```python
from build123d import *

# Parameters (mm, degrees)
STOCK_SHORT_HANDLE_L_1_START = -1
STOCK_SHORT_HANDLE_L_1_DEPTH = 2
FILLET1_R                    = 0.5


# Read off the part's stored shape, not the designer's step: Stock-short-handle_L-1
with BuildPart() as part:
    # Stock-short-handle_L-1 outline → Stock-short-handle_L-1 (new body)
    with BuildSketch(Plane(origin=(0, 0, 0), x_dir=(1, 0, 0), z_dir=(0, 1, 0)).offset(STOCK_SHORT_HANDLE_L_1_START)):
        with BuildLine():
            Line((5, -39.585762407), (-5, -39.585762407))
            Line((-5, -39.585762407), (-5, -43.585762407))
            ThreePointArc((-5, -43.585762407), (-4.810860404, -44.434752748), (-4.279215401, -45.123165398))
            ThreePointArc((-4.279215401, -45.123165398), (-1.203063357, -47.386267754), (2.120784599, -49.266793861))
            ThreePointArc((2.120784599, -49.266793861), (4.058671148, -49.167239185), (5, -47.470414091))
            Line((5, -47.470414091), (5, -39.585762407))
        make_face()
    extrude(amount=STOCK_SHORT_HANDLE_L_1_DEPTH)

    # Fillet1
    fillet1_edges = [part.edges().sort_by_distance(p)[0] for p in [
        (5, 0, 39.585762407),
        (-5, 0, 39.585762407),
    ]]
    fillet(fillet1_edges, radius=FILLET1_R)


solid = part.part
```
Could you check a few things on this model? Use its own coordinates, in mm. Round coordinates to 2 decimals unless told otherwise and drop trailing zeros. Loops run counter-clockwise (first coordinate to the right, second up) from the corner with the lowest first, then second, coordinate; pieces in that order, holes last. Notation, with made-up numbers: (32, 23.5) -> (80, 23.5) arc R5 ccw to (80, 30.5) -> close; hole circle Ø5 at (83, 12.5). An arc over 180 degrees is marked (long way). Put each result on its own line as item: value.
Q1. I want a section at A-A on y = -0.7. Write out the boundary of the cut face in (x, z), and give its area (3 significant figures).
Checks:
outline: (-5, 40.09) arc R0.5 ccw to (-4.5, 39.59) -> (4.5, 39.59) arc R0.5 ccw to (5, 40.09) -> (5, 47.47) arc R2 ccw to (2.12, 49.27) arc R32 ccw to (-4.28, 45.12) arc R2 ccw to (-5, 43.59) -> close
area: 80.9 mm2
Q2. I want a section at B-B on z = 46. Write out the boundary of the cut face in (x, y), and give its area (3 significant figures).
Checks:
outline: (-3.18, -1) -> (5, -1) -> (5, 1) -> (-3.18, 1) -> close
area: 16.4 mm2
Q3. Please list where these lines run through material, in increasing order: line 1 (X direction, y = -0.4, z = 47.5); line 2 (Z direction, x = 2.5, y = 0.7); line 3 (Z direction, x = 4, y = 0.85). Write a range as from..to.
Checks:
line 1: -1.03..5
line 2: 39.59..49.41
line 3: 39.59..49.2
Q4. For pin 1 Ø1.5 at (x, z) = (-2.5, 47) entering from +Y, with a flat end and sliding along its axis, tell me the tip position at first contact or that it passes through.
Checks:
pin 1: y = 1
Q5. I want a section at C-C on x = 0.75. Write out the boundary of the cut face in (y, z), and give its area (3 significant figures).
Checks:
outline: (-1, 39.59) -> (1, 39.59) -> (1, 48.55) -> (-1, 48.55) -> close
area: 17.9 mm2
